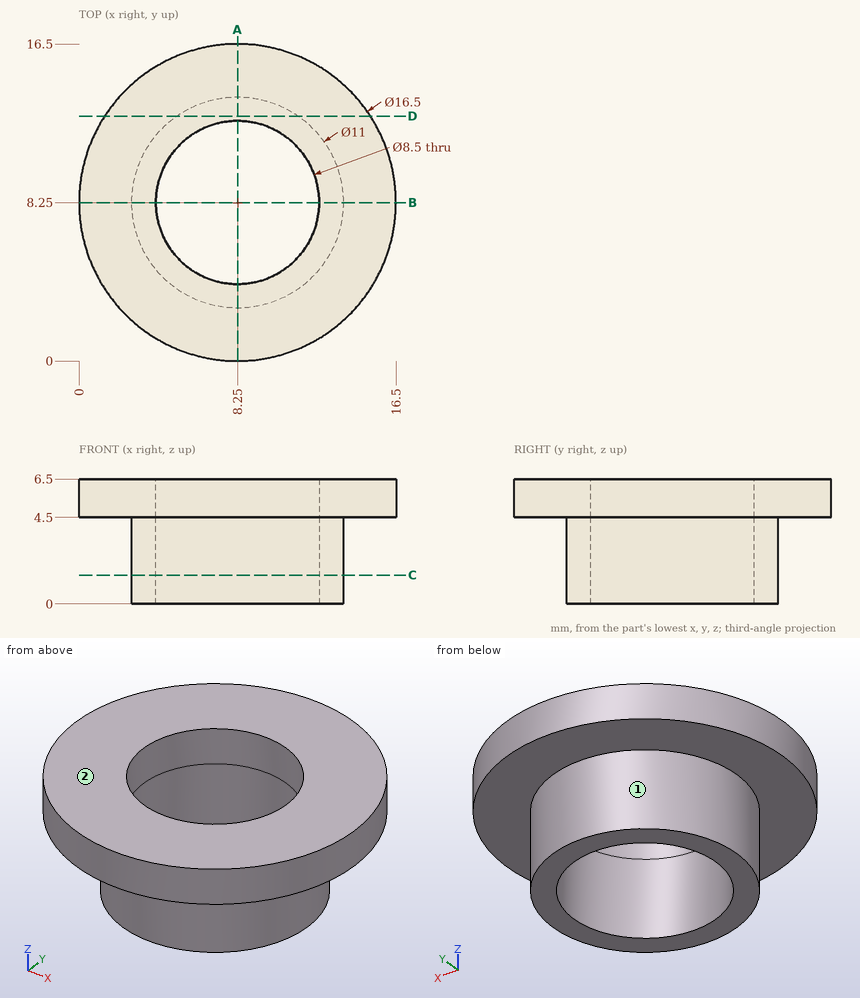
Can you work these out from the drawing? Everything is in mm from the part's minimum corner. A direction names the side the tool comes from. Give positions to 0.01 mm unless a question says otherwise; leave off trailing zeros. Loops run counter-clockwise (first coordinate to the right, second up) from the corner with the lowest first, then second, coordinate; pieces in that order, holes last. Notation, with made-up numbers: M -34,-20.5 L 14,-20.5 A15 cw 14,8.5 Z; hole C 22.5,43.5 d10. An arc over 180 degrees is marked long. Put each result on its own line as item: value. Start each with the question number.
(1) I want a section at A-A on x = 8.25. Please give me the cut outline in (y, z).
(2) I need wall thicknesses on line 1 along X through (y, z) = (8.25, 2.5); line 2 along Y through (x, z) = (8.25, 5.25). Which ranges of each line are inside material? Lowest first, please. Write a range as [from, to].
(3) Will this pin go through, and if not, where does the flat tip stop? pin 1 Ø5 at (x, y) = (8, 7.5) entering from -Z.
(4) For the marked faces 1 and 2, which set-ups out of +Z, -Z, +X, -X, +Y, -Y let a thin tool reach every point of the face, with its end or its side?
(5) I want a section at C-C on z = 1.5. Please give me the cut outline in (x, y).
(6) I want a section at D-D on y = 12.75. Please give me the cut outline in (x, z).
Answer block:
1. outline: M 0,4.5 L 2.75,4.5 L 2.75,0 L 4,0 L 4,6.5 L 0,6.5 Z; M 12.5,0 L 13.75,0 L 13.75,4.5 L 16.5,4.5 L 16.5,6.5 L 12.5,6.5 Z
2. line 1: [2.75, 4], [12.5, 13.75]
2. line 2: [0, 4], [12.5, 16.5]
3. pin 1: through
4. face 1: -Z
4. face 2: +Z, +X, -X, +Y, -Y
5. outline: C 8.25,8.25 d11; hole C 8.25,8.25 d8.5
6. outline: M 1.34,4.5 L 5.09,4.5 L 5.09,0 L 11.41,0 L 11.41,4.5 L 15.16,4.5 L 15.16,6.5 L 1.34,6.5 Z
